Here's how the part is built. I have some questions about the finished solid (model axes, mm). A direction names the side the tool comes from. Round coordinates to 2 decimals unless told otherwise and drop trailing zeros. Order: outer loops, then holes, each group sorted by start corner. A loop starts at its lowest first (then second) coordinate and runs counter-clockwise, first axis right, second up. Notation, with made-up numbers: M 86.25,48.5 L 121.25,48.5 A27 cw 121.25,80.5 Z; hole C -12.75,61.25 d8. An arc over 180 degrees is marked long. Write each question's results on one line, items separated by ' | '. Start each with the question number.
Autodesk Inventor part; units mm, degrees
ref_plane "YZ Plane" through (0, 0, 0) normal (1, 0, 0) x (0, 1, 0)
ref_plane "XZ Plane" through (0, 0, 0) normal (0, 1, 0) x (-1, 0, 0)
ref_plane "XY Plane" through (0, 0, 0) normal (0, 0, 1) x (1, 0, 0)
sketch "Sketch1" plane through (0, 0, 0) normal (0, 0, 1) x (1, 0, 0)
  line L0 (-12.6252, -30.48) -> (-30.48, -12.6252)
  line L1 (-30.48, -12.6252) -> (-30.48, 12.6252)
  line L2 (-30.48, 12.6252) -> (-12.6252, 30.48)
  line L3 (-12.6252, 30.48) -> (12.6252, 30.48)
  line L4 (12.6252, 30.48) -> (30.48, 12.6252)
  line L5 (30.48, 12.6252) -> (30.48, -12.6252)
  line L6 (30.48, -12.6252) -> (12.6252, -30.48)
  line L7 (12.6252, -30.48) -> (-12.6252, -30.48)
  circle A0 centre (0, 0) radius 30.48
  line L8 (28.3719, -11.1385) -> (12.1858, -27.9381)
  line L9 (12.1858, -27.9381) -> (-11.1385, -28.3719)
  line L10 (-11.1385, -28.3719) -> (-27.9381, -12.1858)
  line L11 (-27.9381, -12.1858) -> (-28.3719, 11.1385)
  line L12 (-28.3719, 11.1385) -> (-12.1858, 27.9381)
  line L13 (-12.1858, 27.9381) -> (11.1385, 28.3719)
  line L14 (11.1385, 28.3719) -> (27.9381, 12.1858)
  line L15 (27.9381, 12.1858) -> (28.3719, -11.1385)
  point P0 (0, 0)
  point P1 (0, 30.48)
  dimension "d50" = 60.96
  dimension "d54" = 30.48
extrude "Extrusion1" add sketch "Sketch1" along normal blind 40
sketch "Sketch2" plane through (0, 0, 40) normal (0, 0, 1) x (1, 0, 0)
  line L0 (-43.3633, -42.9193) -> (43.3633, -42.9193)
  line L1 (43.3633, -42.9193) -> (43.3633, 42.9193)
  line L2 (43.3633, 42.9193) -> (-43.3633, 42.9193)
  line L3 (-43.3633, 42.9193) -> (-43.3633, -42.9193)
  line L4 (-43.3633, -42.9193) -> (43.3633, 42.9193) construction
  line L5 (43.3633, -42.9193) -> (-43.3633, 42.9193) construction
  point P0 (0, 0)
extrude "Extrusion2" add sketch "Sketch2" along normal blind 20
fillet "Fillet1" radius 10 4 edges at (43.3633, 42.9193, 50) (43.3633, -42.9193, 50) (-43.3633, 42.9193, 50) (-43.3633, -42.9193, 50)
sketch "Sketch3" plane through (0, 0, 60) normal (0, 0, 1) x (1, 0, 0)
  circle A0 centre (0, 0) radius 19.9292
extrude "Extrusion3" add sketch "Sketch3" along normal blind 5
sketch "Sketch4" plane through (0, 0, 65) normal (0, 0, 1) x (1, 0, 0)
  line L0 (6.9511, -37.5125) -> (-6.9511, -37.5125)
  line L1 (-6.9511, -37.5125) -> (-6.9511, 24.1539)
  line L2 (-6.9511, 24.1539) -> (6.9511, 24.1539)
  line L3 (6.9511, 24.1539) -> (6.9511, -37.5125)
  line L4 (6.9511, -37.5125) -> (-6.9511, 24.1539) construction
  line L5 (-6.9511, -37.5125) -> (6.9511, 24.1539) construction
  point P0 (0, 0)
  point P1 (0, -6.6793)
extrude "Extrusion4" add sketch "Sketch4" along normal blind 15
fillet "Fillet2" radius 15 1 edges at (0, 24.1539, 80)
sketch "Sketch5" plane through (0, 0, 80) normal (0, 0, 1) x (1, 0, 0)
  circle A0 centre (0, 0) radius 5.639
extrude "Extrusion5" cut sketch "Sketch5" against normal blind 20
sketch "Sketch6" plane through (0, 0, 60) normal (0, 0, 1) x (1, 0, 0)
  circle A0 centre (0, 0) radius 5.639
  circle A1 centre (0, 0) radius 5.08
  dimension "d13" = 10.16
extrude "Extrusion6" add sketch "Sketch6" along normal blind 15 contours A1
sketch "Sketch7" plane through (0, 0, 75) normal (0, 0, 1) x (1, 0, 0)
  line L0 (1.4769, -3.2223) -> (-1.4769, -3.2223)
  line L1 (-1.4769, -3.2223) -> (-1.4769, 3.2223)
  line L2 (-1.4769, 3.2223) -> (1.4769, 3.2223)
  line L3 (1.4769, 3.2223) -> (1.4769, -3.2223)
  circle A0 centre (0, 0) radius 5.639
  line L4 (1.4769, -3.2223) -> (-1.4769, 3.2223) construction
  line L5 (-1.4769, -3.2223) -> (1.4769, 3.2223) construction
extrude "Extrusion7" cut sketch "Sketch7" against normal blind 5 contours L0 L1 L2 L3
sketch "Sketch8" plane through (0, 0, 60) normal (0, 0, 1) x (1, 0, 0)
  line L0 (-9.528, 62.156) -> (8.3554, 62.156) construction
  line L1 (8.3554, 62.156) -> (8.3554, 44.2726) construction
  line L2 (8.3554, 44.2726) -> (-9.528, 44.2726) construction
  line L3 (-9.528, 44.2726) -> (-9.528, 62.156) construction
  line L4 (44.1222, 9.3815) -> (61.4167, 9.3815) construction
  line L5 (61.4167, 9.3815) -> (61.4167, -7.913) construction
  line L6 (61.4167, -7.913) -> (44.1222, -7.913) construction
  line L7 (44.1222, -7.913) -> (44.1222, 9.3815) construction
  point P0 (0, 0)
decal "Decal1"
decal "Decal2"
sketch "Sketch9" plane through (-30.48, 12.6252, 0) normal (-1, 0, 0) x (0, -1, 0)
  point P0 (12.6252, 0)
sketch "Sketch10" plane through (0, 0, 60) normal (0, 0, 1) x (1, 0, 0)
  line L0 (-5.7001, 39.3416) -> (5.3375, 39.3416) construction
  line L1 (5.3375, 39.3416) -> (5.3375, 28.3041) construction
  line L2 (5.3375, 28.3041) -> (-5.7001, 28.3041) construction
  line L3 (-5.7001, 28.3041) -> (-5.7001, 39.3416) construction
  line L4 (25.3709, 6.0354) -> (36.3058, 6.0354) construction
  line L5 (36.3058, 6.0354) -> (36.3058, -4.8995) construction
  line L6 (36.3058, -4.8995) -> (25.3709, -4.8995) construction
  line L7 (25.3709, -4.8995) -> (25.3709, 6.0354) construction
  point P0 (0, 0)
decal "Decal3"
decal "Decal4"
properties part number "gabaritna_sklopka"
(1) I'm going to push flat-ended pins straight in: pin 1 Ø6.5 at (x, y) = (15, -2.5) entering from +Z; pin 2 Ø4 at (x, y) = (22.5, -32.5) entering from -Z; pin 3 Ø0.9 at (x, z) = (0.5, 73.5) entering from +Y. Where does each tip first touch, or does it pass through?
(2) On a 3-axis mill with a long thin cutter (end or side, diameter ignored), from which of +Z, -Z, +X, -X, +Y, -Y can I reach the whole of each face in a straight line? I mean faces 5 (the flat face through (30.48, 0, 20)), 6 (the flat face through (0, -30.48, 20)), 7 (the cylindrical face through (-0.661, -5.037, 67.395)). Say none if no direction works.
(3) I want a section at B-B on z = 20.5. Write out the boundary of the cut face in (x, y).
(4) Please list where these lines run through material, in increasing order: line 1 (Y direction, x = 0, z = 68); line 2 (Y direction, x = 0, z = 71); line 3 (Y direction, x = 0, z = 72.75).
(5) I want a section at A-A on y = -22.5. Write out the boundary of the cut face in (x, z), and give its area (3 significant figures).
(6) I want a section at C-C on y = 0. Write out the boundary of the cut face in (x, z).
(7) If we mould it in two halves opening along X, with no side actions, what happens to faces 1 (the flat face through (-6.951, -7, 72)), 2 (the cylindrical face through (40.356, -40.068, 50.14)), 3 (the flat face through (0, 3.222, 73)), 4 (the flat face through (2, 0, 75))? For each: pulls with the +X half, pulls with the -X half, needs draft (parallel to the pull), parting line crosses it, or undercut.
Solutions:
1) pin 1: z = 65 | pin 2: z = 40 | pin 3: y = 21.81
2) face 5: -Z, +X, +Y, -Y | face 6: -Z, +X, -X, -Y | face 7: +Z
3) outline: M -30.48,-12.63 L -12.63,-30.48 L 12.63,-30.48 L 30.48,-12.63 L 30.48,12.63 L 12.63,30.48 L -12.63,30.48 L -30.48,12.63 Z
4) line 1: -37.51 to -5.64, -5.08 to 5.08, 5.64 to 23.85 | line 2: -37.51 to -5.64, -5.08 to -3.22, 3.22 to 5.08, 5.64 to 22.9 | line 3: -37.51 to -5.64, -5.08 to -3.22, 3.22 to 5.08, 5.64 to 22
5) outline: M -43.36,40 L -20.61,40 L -20.61,0 L 20.61,0 L 20.61,40 L 43.36,40 L 43.36,60 L -43.36,60 Z; M -6.95,65 L 6.95,65 L 6.95,80 L -6.95,80 Z | area: 3,590 mm^2
6) outline: M -43.36,40 L -30.48,40 L -30.48,0 L 30.48,0 L 30.48,40 L 43.36,40 L 43.36,60 L 19.93,60 L 19.93,65 L 6.95,65 L 6.95,80 L 5.64,80 L 5.64,60 L 5.08,60 L 5.08,75 L 1.48,75 L 1.48,70 L -1.48,70 L -1.48,75 L -5.08,75 L -5.08,60 L -5.64,60 L -5.64,80 L -6.95,80 L -6.95,65 L -19.93,65 L -19.93,60 L -43.36,60 Z
7) face 1: pulls with the -X half | face 2: pulls with the +X half | face 3: undercut | face 4: undercut
